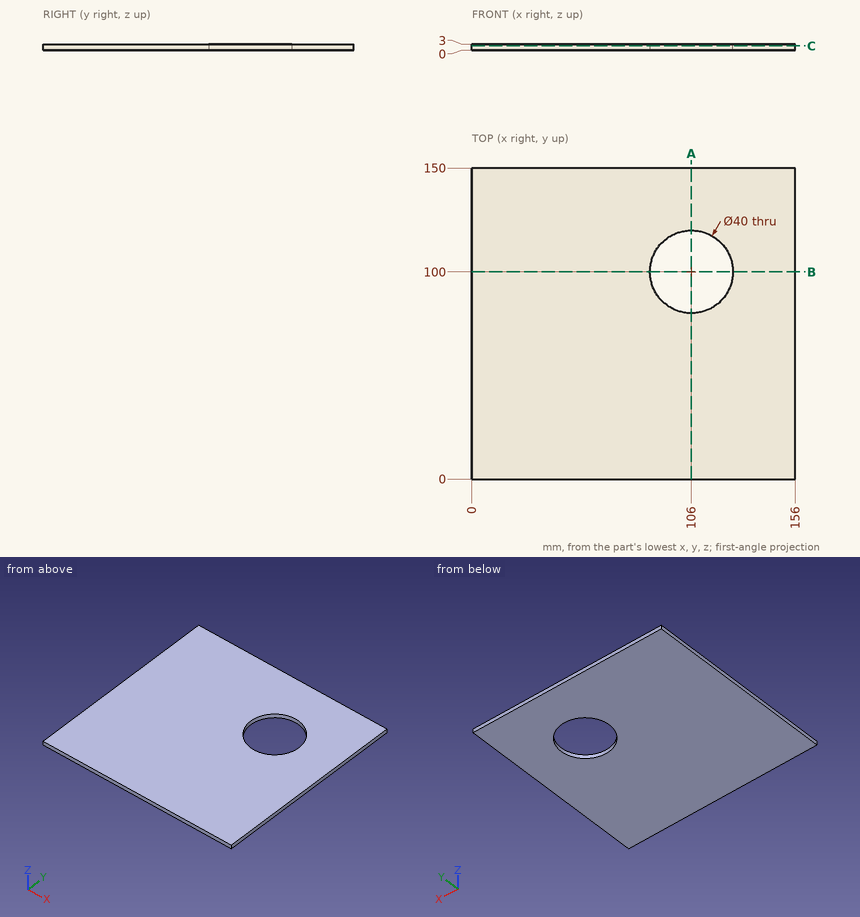
Verification items for this drawing (mm, ordinates from the low corner). Coordinates: 2 decimals unless noted, no trailing zeros. Order: outer loops, then holes, each group sorted by start corner. A loop starts at its lowest first (then second) coordinate and runs counter-clockwise, first axis right, second up. Notation, with made-up numbers: M -3,-35.75 L 41,-35.75 A23 cw 41,-23.75 Z; hole C -38.5,50 d8. An arc over 180 degrees is marked long. Use CSV: the item, a comma, the result in double quotes.
Item 1: Cross-section at C-C on z = 2.05. Record the cut outline in (x, y).
Returned:
outline,"M 0,0 L 156,0 L 156,150 L 0,150 Z; hole C 106,100 d40"
Item 2: Thickness scan on line 1 along Y through (x, z) = (106, 0.95); line 2 along X through (y, z) = (100, 2.05); line 3 along X through (y, z) = (113.5, 1.8). Record the ranges inside material, lowest first.
Returned:
line 1,"y = 0 to 80, 120 to 150"
line 2,"x = 0 to 86, 126 to 156"
line 3,"x = 0 to 91.24, 120.76 to 156"
Item 3: Cross-section at A-A on x = 106. Record the cut outline in (y, z).
Returned:
outline,"M 0,0 L 80,0 L 80,3 L 0,3 Z; M 120,0 L 150,0 L 150,3 L 120,3 Z"
Item 4: Cross-section at B-B on y = 100. Record the cut outline in (x, z), then the cut area to 3 significant figures.
Returned:
outline,"M 0,0 L 86,0 L 86,3 L 0,3 Z; M 126,0 L 156,0 L 156,3 L 126,3 Z"
area,"348 mm2"
